Study the drawing (mm; zero at the part's minimum x, y, z) and answer. A direction names the side the tool comes from. Give positions to 0.01 mm unless a question says otherwise; leave off trailing zeros. Order: outer loops, then holes, each group sorted by start corner. A loop starts at its lowest first (then second) coordinate and runs counter-clockwise, first axis right, second up. Notation, with made-up numbers: (44, -14) - (59, -14) arc R25 cw to (59, 19) - close; hole circle Ø4 at (44, 38). An arc over 180 degrees is marked (long way). Return JSON: item names as keys, results as strings.
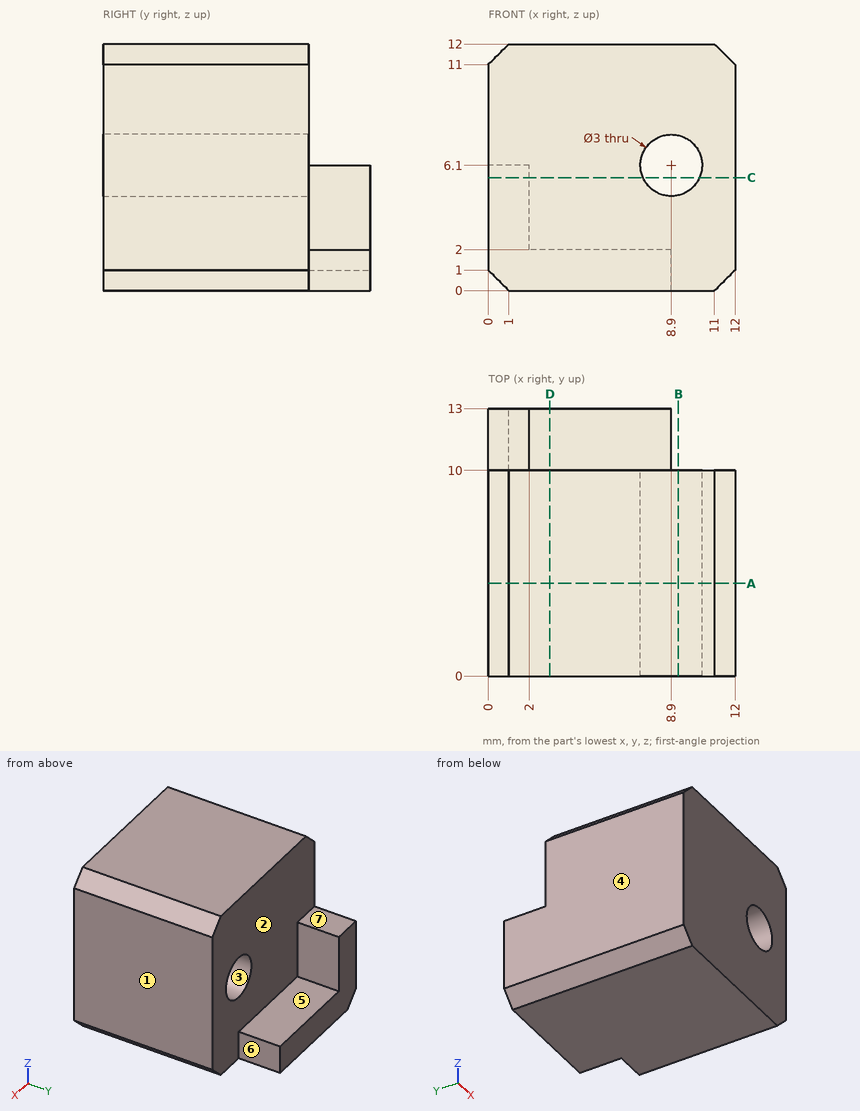
Q1. For the marked faces 5, 6 and 7, determine the directions among +Z, -Z, +X, -X, +Y, -Y from which every point of the face is accessible in a straight line to the end or side of a thin tool.
Values:
{"face 5": "+Z, +X, +Y", "face 6": "+Z, -Z, +X, +Y", "face 7": "+Z, +X, -X, +Y"}
Q2. A cutting plane is placed at A-A (y = 4.5). Write down the section's boundary in (x, z).
Values:
{"outline": "(0, 1) - (1, 0) - (11, 0) - (12, 1) - (12, 11) - (11, 12) - (1, 12) - (0, 11) - close; hole circle Ø3 at (8.9, 6.1)"}
Q3. Determine the mould class of the marked faces 1, 2, 3 and 4 for opening direction X: released by +X, released by -X, zero draft, split by the parting line, or undercut.
Values:
{"face 1": "released by +X", "face 2": "zero draft", "face 3": "undercut", "face 4": "released by -X"}
Q4. A cutting plane is placed at C-C (z = 5.5). Write down the section's boundary in (x, y).
Values:
{"outline": "(0, 0) - (7.53, 0) - (7.53, 10) - (2, 10) - (2, 13) - (0, 13) - close; (10.27, 0) - (12, 0) - (12, 10) - (10.27, 10) - close"}
Q5. Given pin 1 (3.5 mm diameter, centred on x = 3.5, z = 8.5, fed in from +Y); pin 2 (3 mm diameter, centred on x = 2.5, z = 4.5, fed in from +Y); pin 3 (1.5 mm diameter, centred on y = 12, z = 4.5, fed in from +X); pin 4 (1.6 mm diameter, centred on y = 11, z = 1, fed in from +X), each flat-ended and moving along its own axis, determine where each tip first touches the part or whether it passes through.
Values:
{"pin 1": "stops at y = 10", "pin 2": "stops at y = 13", "pin 3": "stops at x = 2", "pin 4": "stops at x = 8.9"}
Q6. Consider L1, parallel to Z at x = 9, y = 3.75; L2, parallel to X at y = 7.75, z = 6.1; L3, parallel to Y at x = 3, z = 3. Determine where each line is inside the solid, lowest interval first.
Values:
{"L1": "z = 0 to 4.6, 7.6 to 12", "L2": "x = 0 to 7.4, 10.4 to 12", "L3": "y = 0 to 10"}
Q7. A cutting plane is placed at D-D (x = 3). Write down the section's boundary in (y, z), and give its area (3 significant figures).
Values:
{"outline": "(0, 0) - (13, 0) - (13, 2) - (10, 2) - (10, 12) - (0, 12) - close", "area": "126 mm²"}
Q8. A cutting plane is placed at B-B (x = 9.25). Write down the section's boundary in (y, z), and give its area (3 significant figures).
Values:
{"outline": "(0, 0) - (10, 0) - (10, 4.64) - (0, 4.64) - close; (0, 7.56) - (10, 7.56) - (10, 12) - (0, 12) - close", "area": "90.8 mm²"}
